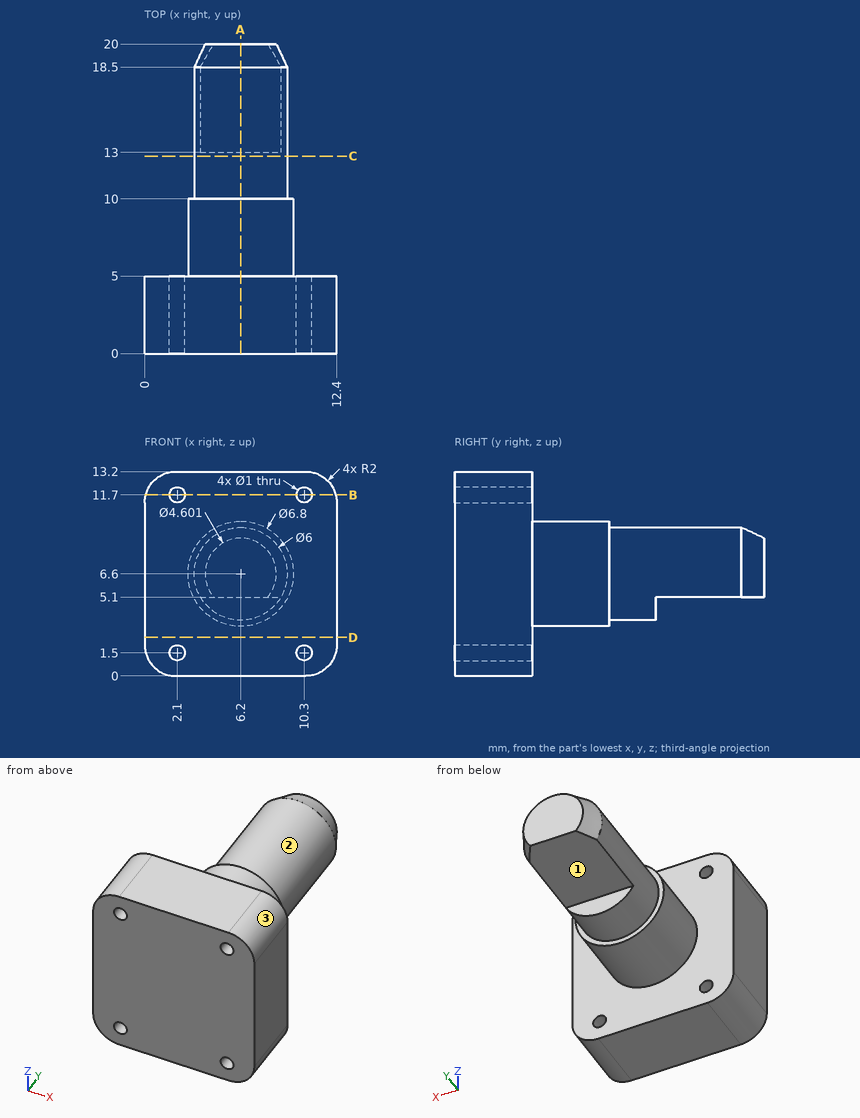
The figure shows three views and two pictorial views of one solid part (mm, origin at its lowest corner). Answer the questions. A direction names the side the tool comes from. Give positions to 0.01 mm unless a question says otherwise; leave off trailing zeros. Write each loop counter-clockwise with the first axis right and the second up, starting at its lowest first coordinate (ties: lowest second). Pieces come first, ordered by that corner, then holes. Notation, with made-up numbers: (71.25, 34.5) -> (89.25, 34.5) arc R27 ccw to (89.25, 60.5) -> close; hole circle Ø10 at (75.25, -39). An arc over 180 degrees is marked (long way). Answer as a JSON object with one key per item and string values.
1) Section D-D on z = 2.5 is taken. Write down the section's boundary in (x, y), then the cut area to 3 significant figures.
Findings below:
{"outline": "(0, 0) -> (12.4, 0) -> (12.4, 5) -> (0, 5) -> close", "area": "62.0 mm^2"}
2) Section A-A on x = 6.2 is taken. Write down the section's boundary in (y, z), then the cut area to 3 significant figures.
Findings below:
{"outline": "(0, 0) -> (5, 0) -> (5, 3.2) -> (10, 3.2) -> (10, 3.6) -> (13, 3.6) -> (13, 5.1) -> (20, 5.1) -> (20, 8.9) -> (18.5, 9.6) -> (10, 9.6) -> (10, 10) -> (5, 10) -> (5, 13.2) -> (0, 13.2) -> close", "area": "149 mm^2"}
3) A tool of negligible diameter and unlimited length cuts with its end or side. For the marked faces 1, 2 and 3, from which of +Z, -Z, +X, -X, +Y, -Y can it reach the whole face along a straight path? Write none if from no direction.
Findings below:
{"face 1": "-Z, +X, -X, +Y", "face 2": "+Y", "face 3": "+Z, +X, +Y, -Y"}
4) Section C-C on y = 12.75 is taken. Write down the section's boundary in (x, z), then the cut area to 3 significant figures.
Findings below:
{"outline": "circle Ø6 at (6.2, 6.6)", "area": "28.3 mm^2"}
5) Section B-B on z = 11.7 is taken. Write down the section's boundary in (x, y), then the cut area to 3 significant figures.
Findings below:
{"outline": "(0.06, 0) -> (1.6, 0) -> (1.6, 5) -> (0.06, 5) -> close; (2.6, 0) -> (9.8, 0) -> (9.8, 5) -> (2.6, 5) -> close; (10.8, 0) -> (12.34, 0) -> (12.34, 5) -> (10.8, 5) -> close", "area": "51.4 mm^2"}
6) Flat-ended cylindrical pins translate along their axes: pin 1 Ø1.7 at (x, z) = (6, 4) entering from +Y; pin 2 Ø4 at (x, y) = (6.5, 7.5) entering from +Z; pin 3 Ø1.6 at (x, y) = (7, 15.5) entering from -Z. Find the tip coordinate at first contact, or state that the pin passes through.
Findings below:
{"pin 1": "stops at y = 13", "pin 2": "stops at z = 10", "pin 3": "stops at z = 5.1"}
7) Straight lines are drawn through the part: probe 1 along X at (y, z) = (4.05, 1.5); probe 2 along Z at (x, y) = (2, 4); probe 3 along Y at (x, z) = (1.25, 1.5). For each, find the intervals that lie inside material, in ascending order. Write a range as from..to.
Findings below:
{"probe 1": "x = 0.06..1.6, 2.6..9.8, 10.8..12.34", "probe 2": "z = 0..1.01, 1.99..11.21, 12.19..13.2", "probe 3": "y = 0..5"}
